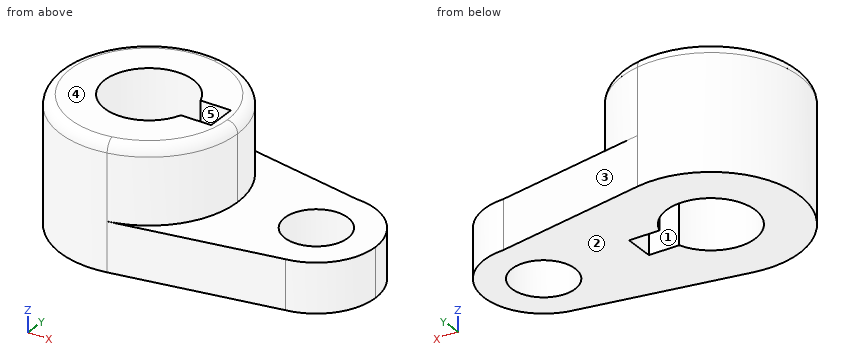
from build123d import *

# Parameters (mm, degrees)
F1_DEPTH = 40.2336
F2_DEPTH = 15.7734
F3_R     = 3.302


with BuildPart() as f1:
    # F0 (on Top) → F1 (new body)
    with BuildSketch(Plane.XY):
        with BuildLine():
            ThreePointArc((-30.217025, -28.124403), (-13.351678, -18.33162), (-6.696585, 0))
            ThreePointArc((-6.696585, 0), (-13.314561, 18.287146), (-30.103039, 28.103679))
            ThreePointArc((-30.103039, 28.103679), (-63.846526, 0.057927), (-30.217025, -28.124403))
        make_face()
        with BuildLine():
            Line((-12.062577, 4.826), (-12.062577, 0))
            Line((-12.062577, 0), (-12.062577, -4.826))
            Line((-12.062577, -4.826), (-21.82382, -4.826))
            ThreePointArc((-21.82382, -4.826), (-49.559085, 0), (-21.82382, 4.826))
            Line((-21.82382, 4.826), (-12.062577, 4.826))
        make_face(mode=Mode.SUBTRACT)
    extrude(amount=F1_DEPTH)

    # F0 (on Top) → F2 (join)
    with BuildSketch(Plane.XY):
        with BuildLine():
            Line((-0.346585, 0), (-6.696585, 0))
            ThreePointArc((-6.696585, 0), (-13.351678, -18.33162), (-30.217025, -28.124403))
            Line((-30.217025, -28.124403), (21.158081, -18.891191))
            ThreePointArc((21.158081, -18.891191), (6.130804, -14.311951), (-0.346585, 0))
        make_face()
        with BuildLine():
            ThreePointArc((-30.103039, 28.103679), (-13.314561, 18.287146), (-6.696585, 0))
            Line((-6.696585, 0), (-0.346585, 0))
            ThreePointArc((-0.346585, 0), (5.393624, 13.629085), (19.154934, 19.044648))
            Line((19.154934, 19.044648), (-30.103039, 28.103679))
        make_face()
        with BuildLine():
            ThreePointArc((19.154934, 19.044648), (5.393624, 13.629085), (-0.346585, 0))
            ThreePointArc((-0.346585, 0), (6.130804, -14.311951), (21.158081, -18.891191))
            ThreePointArc((21.158081, -18.891191), (33.015366, -12.572611), (37.753415, 0))
            ThreePointArc((37.753415, 0), (32.3325, 13.309791), (19.154934, 19.044648))
        make_face()
        with BuildLine():
            ThreePointArc((28.863415, 0), (18.703415, -10.16), (8.543415, 0))
            ThreePointArc((8.543415, 0), (18.703415, 10.16), (28.863415, 0))
        make_face(mode=Mode.SUBTRACT)
    extrude(amount=F2_DEPTH)

    # F3
    f3_edges = [f1.edges().sort_by_distance(p)[0] for p in [
        (-40.326145, 28.124403, 40.2336),
    ]]
    fillet(f3_edges, radius=F3_R)


solid = f1.part
Part model, mm, in its own coordinate system. Face numbers are marked on the shaded views. A direction names the side the tool comes from. Give positions to 0.01 mm unless a question says otherwise; leave off trailing zeros. Write each loop counter-clockwise with the first axis right and the second up, starting at its lowest first coordinate (ties: lowest second). Pieces come first, ordered by that corner, then holes.
1) Probe L1, parallel to Y at x = -34.5, z = 35; L2, parallel to Z at x = -12.5, y = -17.5; L3, parallel to Y at x = -29, z = 18. List the from-to ranges inside material, lowest first.
Resolved:
L1: y = -28.56 to -14.27, 14.27 to 28.56
L2: z = 0 to 15.77
L3: y = -27.88 to -12.84, 12.84 to 27.88
2) Which spindle directions (+Z, -Z, +X, -X, +Y, -Y) get a long thin tool onto all of the face, cutting with end or side? Do the marked faces 1 and 2. Say none if no direction does.
Resolved:
face 1: +Z, -Z
face 2: -Z, +X, -X, +Y, -Y
3) Cut at A-A on z = 10. State how many separate pieces and enclosed holes the cut face has, then the cut area to 3 significant figures.
Resolved:
separate pieces: 1
enclosed holes: 2
area: 3,400 mm2
4) Pin check, flat tips, straight feed: pin 1 (8 mm diameter, centred on x = 13.5, y = -16.5, fed in from -Z); pin 2 (16.5 mm diameter, centred on x = 18.7, y = 0, fed in from -Z); pin 3 (5 mm diameter, centred on y = -2.5, z = 14.5, fed in from -X); pin 4 (10 mm diameter, centred on x = 26.5, z = 6, fed in from -Y). Stop position of each tip, or through.
Resolved:
pin 1: stops at z = 0
pin 2: passes through
pin 3: stops at x = -63.85
pin 4: stops at y = -18.84
5) Cut at B-B on x = 10.5. Write the cut outline in (y, z).
Resolved:
outline: (-20.81, 0) - (-5.99, 0) - (-5.99, 15.77) - (-20.81, 15.77) - close; (5.99, 0) - (20.64, 0) - (20.64, 15.77) - (5.99, 15.77) - close
6) Two-plate mould, pull along Y, no slides. Class the marked faces 3, 4 and 5: released by +Y, released by -Y, zero draft, split by the parting line, or undercut.
Resolved:
face 3: released by +Y
face 4: zero draft
face 5: undercut
